```python
from build123d import *

# Parameters (mm, degrees)
SKETCH1_R           = 45
BOSS_EXTRUDE1_DEPTH = 5


with BuildPart() as part:
    # Sketch1 → Boss-Extrude1 (new body)
    with BuildSketch(Plane.XY):
        Polygon((-230.557942617, -6.721028691), (-168.142249758, -157.405840896), (-158.242754822, -167.305335833), (-7.557942617, -229.721028692), (6.442057383, -229.721028692), (157.126869588, -167.305335833), (167.026364524, -157.405840896), (229.442057383, -6.721028691), (229.442057383, 7.278971309), (167.026364524, 157.963783513), (157.126869588, 167.86327845), (6.442057383, 230.278971308), (-7.557942617, 230.278971308), (-158.242754822, 167.86327845), (-168.142249758, 157.963783513), (-230.557942617, 7.278971308), align=None)
        Circle(SKETCH1_R, mode=Mode.SUBTRACT)
    extrude(amount=BOSS_EXTRUDE1_DEPTH)


solid = part.part
```
Geometry: final body of the model. Coordinates: model frame, mm. Round coordinates to 2 decimals unless told otherwise and drop trailing zeros. Write each loop counter-clockwise with the first axis right and the second up, starting at its lowest first coordinate (ties: lowest second). Pieces come first, ordered by that corner, then holes. Notation, with made-up numbers: (-15, -14) -> (20, -14) arc R16 ccw to (20, 11) -> close; hole circle Ø4 at (35.5, 51.25). An arc over 180 degrees is marked (long way). Use CSV: the item, a comma, the result in double quotes. Start each with the question number.
Q1. Section D-D (x = 150). Return loops of the section in (y, z), plus the area to 3 significant figures.
Q2. Line query: L1, parallel to Y at x = 0, z = 1.9; L2, parallel to X at y = -15, z = 3.45; L3, parallel to X at y = -37, z = 4.8. Output: solid intervals per line, ascending.
Q3. Section B-B (x = 0). Return loops of the section in (y, z), plus the area to 3 significant figures.
Q4. First-contact query: pin 1 Ø10 at (x, y) = (-171, -17.5) entering from -Z. Flat tip, straight axial feed; report the tip coordinate or a pass-through.
Q5. Section C-C (z = 3.55). Return loops of the section in (x, y).
Q6. Pull-direction query (X, two-part tool) for faces 1 (the face through (-83.955, -198.076, 2.465)), 2 (the face through (47, 3, 0)), 3 (the face through (20.765, -39.923, 2.465)); classes: pulls with the +X half, pulls with the -X half, needs draft (parallel to the pull), parting line crosses it, or undercut.
Q7. Section A-A (y = 0). Return loops of the section in (x, z).
Result sheet:
1,outline,"(-170.26, 0) -> (170.82, 0) -> (170.82, 5) -> (-170.26, 5) -> close"
1,area,"1,710 mm²"
2,L1,"-229.72 to -45, 45 to 230.28"
2,L2,"-227.13 to -42.43, 42.43 to 226.01"
2,L3,"-218.02 to -25.61, 25.61 to 216.9"
3,outline,"(-229.72, 0) -> (-45, 0) -> (-45, 5) -> (-229.72, 5) -> close; (45, 0) -> (230.28, 0) -> (230.28, 5) -> (45, 5) -> close"
3,area,"1,850 mm²"
4,pin 1,"z = 0"
5,outline,"(-230.56, -6.72) -> (-168.14, -157.41) -> (-158.24, -167.31) -> (-7.56, -229.72) -> (6.44, -229.72) -> (157.13, -167.31) -> (167.03, -157.41) -> (229.44, -6.72) -> (229.44, 7.28) -> (167.03, 157.96) -> (157.13, 167.86) -> (6.44, 230.28) -> (-7.56, 230.28) -> (-158.24, 167.86) -> (-168.14, 157.96) -> (-230.56, 7.28) -> close; hole circle Ø90 at (0, 0)"
6,face 1,"pulls with the -X half"
6,face 2,"needs draft"
6,face 3,"undercut"
7,outline,"(-230.56, 0) -> (-45, 0) -> (-45, 5) -> (-230.56, 5) -> close; (45, 0) -> (229.44, 0) -> (229.44, 5) -> (45, 5) -> close"
